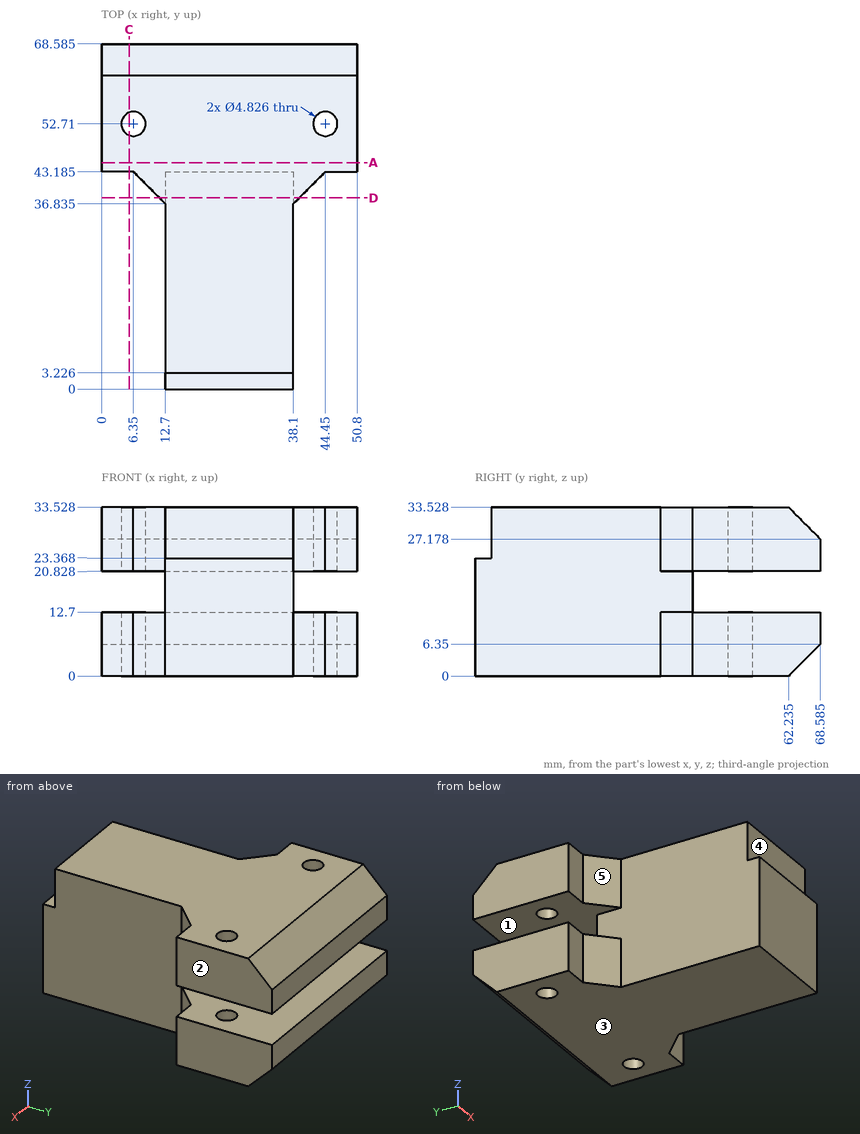
The figure shows three views and two pictorial views of one solid part (mm, origin at its lowest corner). Answer the questions. A direction names the side the tool comes from. Give positions to 0.01 mm unless a question says otherwise; leave off trailing zeros. Order: outer loops, then holes, each group sorted by start corner. A loop starts at its lowest first (then second) coordinate and runs counter-clockwise, first axis right, second up. Notation, with made-up numbers: (31, 15) -> (46, 15) arc R23 ccw to (46, 51) -> close; hole circle Ø2 at (59, 76). An arc over 180 degrees is marked (long way). One line per item, written item: value.
1) Find section A-A, the plane y = 45. Determine the outline of the cut face in (x, z).
Reported:
outline: (0, 0) -> (50.8, 0) -> (50.8, 12.7) -> (0, 12.7) -> close; (0, 20.83) -> (50.8, 20.83) -> (50.8, 33.53) -> (0, 33.53) -> close
2) Determine the mould class of the marked faces 1, 2 and 3 for opening direction Z: pulls with the +Z half, pulls with the -Z half, needs draft (parallel to the pull), parting line crosses it, or undercut.
Reported:
face 1: undercut
face 2: needs draft
face 3: pulls with the -Z half
3) Flat-ended cylindrical pins translate along their axes: P1, Ø8, axis at x = 6.5, z = 21.5, coming from the -Y side (1 decimal); P2, Ø17, axis at y = 32, z = 20, coming from the -X side (1 decimal); P3, Ø8, axis at x = 25.5, z = 30.5, coming from the -Y side; P4, Ø4.5, axis at x = 6.35, y = 52.71, coming from the -Z side. Find the tip coordinate at first contact, or state that the pin passes through.
Reported:
P1: stops at y = 39
P2: stops at x = 9.1
P3: stops at y = 3.23
P4: passes through
4) A tool of negligible diameter and unlimited length cuts with its end or side. For the marked faces 4 and 5, from which of +Z, -Z, +X, -X, +Y, -Y can it reach the whole face along a straight path? Write none if from no direction.
Reported:
face 4: +Z, +X, -X, -Y
face 5: +Z, -Z, -X, -Y
5) Find the intervals of material crossed by line 1 (Z direction, x = 24.5, y = 62); line 2 (X direction, y = 14.5, z = 26); line 3 (Y direction, x = 6, z = 6) (1 decimal), in increasing order.
Reported:
line 1: z = 0 to 12.7, 20.83 to 33.53
line 2: x = 12.7 to 38.1
line 3: y = 43.2 to 50.3, 55.1 to 68.2
6) Find section C-C, the plane x = 5.5. Count the separate pieces of the cut face and the enclosed holes in it, plus the area to 3 significant figures.
Reported:
separate pieces: 4
enclosed holes: 0
area: 490 mm^2
7) Find section D-D, the plane y = 38. Determine the outline of the cut face in (x, z) (1 decimal), plus the area to 3 significant figures.
Reported:
outline: (11.5, 0) -> (39.3, 0) -> (39.3, 12.7) -> (38.1, 12.7) -> (38.1, 20.8) -> (39.3, 20.8) -> (39.3, 33.5) -> (11.5, 33.5) -> (11.5, 20.8) -> (12.7, 20.8) -> (12.7, 12.7) -> (11.5, 12.7) -> close
area: 911 mm^2
